Autodesk Inventor part; units mm, degrees
ref_plane "Work Plane3" through (54.9275, 0, 88.9) normal (1, 0, 0) x (0, 0, -1)
ref_plane "YZ Plane" through (0, 0, 0) normal (1, 0, 0) x (0, 1, 0)
ref_plane "XZ Plane" through (0, 0, 0) normal (0, 1, 0) x (-1, 0, 0)
sketch "Sketch1" plane through (0, 0, 0) normal (0, 0, 1) x (1, 0, 0)
  line L0 (0, 0) -> (109.855, 0)
  line L1 (109.855, 0) -> (109.855, -1.5875)
  line L2 (109.855, -1.5875) -> (0, -1.5875)
  line L3 (0, -1.5875) -> (0, 0)
  line L4 (109.855, 0) -> (108.2675, 0)
  line L5 (108.2675, 0) -> (108.2675, -153.2655)
  line L6 (108.2675, -153.2655) -> (109.855, -153.2655)
  line L7 (109.855, -153.2655) -> (109.855, 0)
  line L8 (0, 0) -> (1.5875, 0)
  line L9 (1.5875, 0) -> (1.5875, -153.2655)
  line L10 (1.5875, -153.2655) -> (0, -153.2655)
  line L11 (0, -153.2655) -> (0, 0)
  line L12 (0, -151.678) -> (25.4, -151.678) construction
  line L13 (1.5875, -153.2655) -> (38.1, -153.2655) construction
  line L14 (0, -153.2655) -> (-6.4677, -177.4031)
  line L15 (1.5875, -153.2655) -> (-4.9865, -177.8)
  line L16 (-6.4677, -177.4031) -> (-4.9865, -177.8)
  line L17 (54.9275, 0) -> (54.9275, -59.745)
  line L18 (109.855, -153.2655) -> (116.3227, -177.4031)
  line L19 (108.2675, -153.2655) -> (114.8415, -177.8)
  line L20 (116.3227, -177.4031) -> (114.8415, -177.8)
  dimension "d1" = 1.5875
  dimension "d2" = 1.5875
  dimension "d3" = 153.2655
  dimension "d5" = 153.2655
  dimension "d6" = 1.5875
  dimension "d13" = 1.5875
  dimension "d15" = 106.68
  dimension "d28" = 0
  dimension "d29" = 75
  dimension "d30" = 25.4
  dimension "d31" = 53.34
  dimension "d32" = 177.8
  dimension "d33" = 24.5345
extrude "Extrusion4" add sketch "Sketch1" along normal blind 88.9 contours L0 L9 L2 L3 | L0 L17 L2 L9 | L0 L5 L2 L17 | L0 L1 L2 L5
extrude "Extrusion5" add sketch "Sketch1" along normal blind 67.31 contours L0 L9 L2 L3 | L2 L9 L10 L11 | L10 L15 L16 L14 | L0 L1 L2 L5 | L2 L7 L6 L5 | L6 L18 L20 L19
ref_plane "Work Plane3" through (54.9275, 0, 88.9) normal (1, 0, 0) x (0, 0, -1)
sketch "Sketch4" plane through (0, 0, 0) normal (0, 1, 0) x (1, 0, 0)
  line L0 (0, -88.9) -> (109.855, -88.9)
  line L1 (23.1775, -88.9) -> (86.6775, -88.9)
  line L2 (86.6775, -88.9) -> (86.6775, -19.05)
  line L3 (86.6775, -19.05) -> (23.1775, -19.05)
  line L4 (23.1775, -19.05) -> (23.1775, -88.9)
  line L5 (109.855, 0) -> (109.855, -88.9)
  line L6 (0, 0) -> (0, -88.9)
  line L7 (109.855, 0) -> (0, 0)
  dimension "d42" = 109.855
  dimension "d43" = 63.5
  dimension "d44" = 23.1775
  dimension "d45" = 19.05
extrude "Extrusion7" cut sketch "Sketch4" against normal through all contours L4 L3 L2 L0
equation "\"d2\" = d1"
equation "\"d3\" = d5"
equation "\"d6\" = d4"
equation "\"d13\" = d2"
equation "\"d44\" = -0.5 * d43 + 0.5 * d42"
equation "\"d4\" = d2"
properties part number "U-Part Gen 2"
Here's how the part is built. I have some questions about the finished solid (model axes, mm). A direction names the side the tool comes from. Coordinates: 2 decimals unless noted, no trailing zeros. Order: outer loops, then holes, each group sorted by start corner. A loop starts at its lowest first (then second) coordinate and runs counter-clockwise, first axis right, second up. Notation, with made-up numbers: M 25.25,48 L 65.25,48 A30 cw 65.25,72 Z; hole C 4.25,80.5 d3. An arc over 180 degrees is marked long. Answer as CSV lines item,"result". Start each with the question number.
1. We'd pull the mould along X, two halves only. Please class faces 4 (the flat face through (54, 0, 14)), 5 (the flat face through (56, -1.588, 14)), 6 (the flat face through (113, -165, 33)): released by +X, released by -X, zero draft, split by the parting line, or undercut.
2. On a 3-axis mill with a long thin cutter (end or side, diameter ignored), from which of +Z, -Z, +X, -X, +Y, -Y can I reach the whole of each face in a straight line? I mean faces 1 (the flat face through (109.855, -76, 34)), 2 (the flat face through (1, -89, 67.31)), 3 (the flat face through (0, -78, 34)). Say none if no direction works.
3. I want a section at A-A, the plane z = 48. Write out the boundary of the cut face in (x, y) (1 decimal).
4. For pin 1 (0.5 mm diameter, centred on y = -1, z = 66.5, fed in from +X) (3 decimals); pin 2 (9 mm diameter, centred on x = 113.5, y = -100.5, fed in from +Z); pin 3 (0.8 mm diameter, centred on x = 65, y = -1, fed in from +Z), each with a flat end and sliding along its axis, tell me the tip position at first contact or that it passes through.
5. I want a section at B-B, the plane y = -133.5. Write out the boundary of the cut face in (x, z) (1 decimal), and give its area (3 significant figures).
6. I want a section at D-D, the plane x = 11. Write out the boundary of the cut face in (y, z).
7. I need wall thicknesses on line 1 (X direction, y = -30, z = 12) (1 decimal); line 2 (Y direction, x = 97, z = 50); line 3 (X direction, y = -159.5, z = 7). Which ranges of each line are inside material? Lowest first, please. Write a range as [from, to].
8. I want a section at C-C, the plane z = 80. Write out the boundary of the cut face in (x, y) (1 decimal), and give its area (3 significant figures).
Recorded:
1,face 4,"zero draft"
1,face 5,"undercut"
1,face 6,"released by +X"
2,face 1,"+Z, -Z, +X, +Y"
2,face 2,"+Z, +X, -X, -Y"
2,face 3,"+Z, -Z, -X, +Y"
3,outline,"M -6.5,-177.4 L -5,-177.8 L 1.6,-153.3 L 1.6,-1.6 L 23.2,-1.6 L 23.2,0 L 0,0 L 0,-153.3 Z; M 86.7,-1.6 L 108.3,-1.6 L 108.3,-153.3 L 114.8,-177.8 L 116.3,-177.4 L 109.9,-153.3 L 109.9,0 L 86.7,0 Z"
4,pin 1,"stops at x = 109.855"
4,pin 2,"stops at z = 67.31"
4,pin 3,"stops at z = 19.05"
5,outline,"M 0,0 L 1.6,0 L 1.6,67.3 L 0,67.3 Z; M 108.3,0 L 109.9,0 L 109.9,67.3 L 108.3,67.3 Z"
5,area,"214 mm2"
6,outline,"M -1.59,0 L 0,0 L 0,88.9 L -1.59,88.9 Z"
7,line 1,"x = [0, 1.6], [108.3, 109.9]"
7,line 2,"y = [-1.59, 0]"
7,line 3,"x = [-1.67, -0.08], [109.94, 111.53]"
8,outline,"M 0,-1.6 L 23.2,-1.6 L 23.2,0 L 0,0 Z; M 86.7,-1.6 L 109.9,-1.6 L 109.9,0 L 86.7,0 Z"
8,area,"73.6 mm2"
